Part model, mm, in its own coordinate system. Face numbers are marked on the shaded views. A direction names the side the tool comes from. Round coordinates to 2 decimals unless told otherwise and drop trailing zeros. Loops run counter-clockwise (first coordinate to the right, second up) from the corner with the lowest first, then second, coordinate; pieces in that order, holes last. Notation, with made-up numbers: M -12,-34 L 37,-34 A21 cw 37,-18 Z; hole C 84,4 d3. An arc over 180 degrees is marked long. Answer as CSV lines item,"result". Start each with the question number.
Item 1: Band-saw the part on A-A (y = 47). Give the cut face in (x, z).
Item 2: Which spindle directions (+Z, -Z, +X, -X, +Y, -Y) get a long thin tool onto all of the face, cutting with end or side? Do the marked faces 1, 2 and 3. Say none if no direction does.
Item 3: Band-saw the part on C-C (z = 4.25). Count the separate pieces of the cut face and the enclosed holes in it, and give its area (3 significant figures).
Item 4: Drop flat-ended pins along their axis: pin 1 Ø1.5 at (y, z) = (46.5, 3.5) entering from -X; pin 2 Ø0.8 at (x, y) = (-45, -0.5) entering from +Z; pin 3 Ø0.5 at (y, z) = (48.5, 4) entering from -X; pin 4 Ø1.8 at (x, y) = (-58.66, 30) entering from +Z. Give the stop position or say it passes through.
Item 5: Mould opens along X. For the marked faces 4, 5 and 6 say: pulls with the +X half, pulls with the -X half, needs draft (parallel to the pull), parting line crosses it, or undercut.
Item 6: Wall check: line 1 (Y direction, x = -50, z = 1.25); line 2 (X direction, y = 20, z = 2.7); line 3 (X direction, y = 11.5, z = 2.05). Give the ranges that are in metal, low to high.
Item 7: Band-saw the part on B-B (y = 20). Give the cut face in (x, z).
Autodesk Fusion 360 part; units mm, degrees
sketch "Sketch3" plane through (0, 0, 0) normal (0, 0, 1) x (1, 0, 0)
  circle A0 centre (-50, 25) radius 27.5
  line L0 (-40.5, 45) -> (-40.5, 60)
  line L1 (-59.5, 60) -> (-59.5, 45)
  line L2 (-50, 25) -> (-50, 55)
  circle A1 centre (-50, 25) radius 16.25
  spline S0 degree 2 poles (-59.5, 45) (-50.3564, 40) (-40.5, 45) knots 0 0 0 2.042764 2.042764 2.042764 weights 1 3 1
  dimension "d9" = 55
  dimension "d10" = 32.5
extrude "Extrude3" add sketch "Sketch3" along normal blind 5 contours A0 L0 L1 L2 A1 S0 | A0 L0 L2 S0 | A0 L1 L2 S0 | A1
sketch "Sketch4" plane through (0, 0, 5) normal (0, 0, 1) x (-1, 0, 0)
  circle A0 centre (50, -25) radius 27.5
  line L0 (50, -25) -> (50, -61)
  line L1 (59.5, -45) -> (59.5, -62)
  line L2 (40.5, -62) -> (40.5, -45)
  circle A1 centre (50, -25) radius 16.25
  spline S0 degree 2 poles (59.5, -45) (50, -40) (40.5, -45) knots 0 0 0 2.04267 2.04267 2.04267 weights 1 3 1
  line L3 (82.2534, -45.4687) -> (66.0855, -40.2154)
  spline S1 degree 2 poles (71.9568, -22.1453) (64.2658, -29.6353) (66.0855, -40.2154) knots 0 0 0 2.04267 2.04267 2.04267 weights 1 3 1
  line L4 (71.9568, -22.1453) -> (88.1248, -27.3986)
  line L5 (50, -25) -> (84.238, -36.1246)
  line L6 (79.4337, -0.6503) -> (69.4414, -14.4036)
  spline S2 degree 2 poles (54.07, -3.2357) (58.8168, -12.8647) (69.4414, -14.4036) knots 0 0 0 2.04267 2.04267 2.04267 weights 1 3 1
  line L7 (54.07, -3.2357) -> (64.0624, 10.5176)
  line L8 (50, -25) -> (71.1603, 4.1246)
  line L9 (35.9376, 10.5176) -> (45.93, -3.2357)
  spline S3 degree 2 poles (30.5586, -14.4036) (41.1832, -12.8647) (45.93, -3.2357) knots 0 0 0 2.04267 2.04267 2.04267 weights 1 3 1
  line L10 (30.5586, -14.4036) -> (20.5663, -0.6503)
  line L11 (50, -25) -> (28.8397, 4.1246)
  line L12 (11.8752, -27.3986) -> (28.0432, -22.1453)
  spline S4 degree 2 poles (33.9145, -40.2154) (35.7342, -29.6353) (28.0432, -22.1453) knots 0 0 0 2.04267 2.04267 2.04267 weights 1 3 1
  line L13 (33.9145, -40.2154) -> (17.7466, -45.4687)
  line L14 (50, -25) -> (15.762, -36.1246)
  dimension "d14" = 32.5
  dimension "d21" = 360
extrude "Extrude4" cut sketch "Sketch4" against normal blind 30 contours A0 S1 L4 L5 | A0 L3 S1 L5 | A0 L6 S2 L8 | A0 S2 L7 L8 | A0 L0 L1 S0 | A0 L0 L2 S0 | A0 L12 S4 L14 | A0 S4 L13 L14 | A0 L9 S3 L11 | A0 S3 L10 L11
sketch "Sketch5" plane through (0, 0, 5) normal (0, 0, 1) x (-1, 0, 0)
  line L0 (71.9568, -22.1453) -> (77.4796, -23.9398)
  arc A0 (77.4796, -23.9398) -> (72.8546, -9.7057) centre (50, -25) ccw
  line L1 (72.8546, -9.7057) -> (69.4414, -14.4036)
  spline S0 degree 2 poles (69.4414, -14.4036) (58.8168, -12.8647) (54.07, -3.2357) knots -2.04267 -2.04267 -2.04267 0 0 0 weights 1 3 1
  line L2 (54.07, -3.2357) -> (57.4833, 1.4622)
  arc A1 (57.4833, 1.4622) -> (42.5167, 1.4622) centre (50, -25) ccw
  line L3 (42.5167, 1.4622) -> (45.93, -3.2357)
  spline S1 degree 2 poles (45.93, -3.2357) (41.1832, -12.8647) (30.5586, -14.4036) knots -2.04267 -2.04267 -2.04267 0 0 0 weights 1 3 1
  line L4 (30.5586, -14.4036) -> (27.1454, -9.7057)
  arc A2 (27.1454, -9.7057) -> (22.5204, -23.9398) centre (50, -25) ccw
  line L5 (22.5204, -23.9398) -> (28.0432, -22.1453)
  spline S2 degree 2 poles (28.0432, -22.1453) (35.7342, -29.6353) (33.9145, -40.2154) knots -2.04267 -2.04267 -2.04267 0 0 0 weights 1 3 1
  line L6 (33.9145, -40.2154) -> (28.3918, -42.0098)
  arc A3 (28.3918, -42.0098) -> (40.5, -50.807) centre (50, -25) ccw
  line L7 (40.5, -50.807) -> (40.5, -45)
  spline S3 degree 2 poles (40.5, -45) (50, -40) (59.5, -45) knots -2.04267 -2.04267 -2.04267 0 0 0 weights 1 3 1
  line L8 (59.5, -45) -> (59.5, -50.807)
  arc A4 (59.5, -50.807) -> (71.6082, -42.0098) centre (50, -25) ccw
  line L9 (71.6082, -42.0098) -> (66.0855, -40.2154)
  spline S4 degree 2 poles (66.0855, -40.2154) (64.2658, -29.6353) (71.9568, -22.1453) knots -2.04267 -2.04267 -2.04267 0 0 0 weights 1 3 1
  circle A5 centre (50, -25) radius 10
  circle A6 centre (50, -35) radius 1.5
  circle A7 centre (58.6603, -30) radius 1.5
  circle A8 centre (58.6603, -20) radius 1.5
  circle A9 centre (50, -15) radius 1.5
  circle A10 centre (41.3397, -20) radius 1.5
  circle A11 centre (41.3397, -30) radius 1.5
  circle A12 centre (50, -25) radius 6
  line L10 (50, -25) -> (33.8359, -47.248)
  circle A13 centre (35.5881, -44.8363) radius 1.5
  circle A14 centre (64.4119, -44.8363) radius 1.5
  circle A15 centre (73.319, -17.4232) radius 1.5
  circle A16 centre (50, -0.481) radius 1.5
  circle A17 centre (26.681, -17.4232) radius 1.5
  dimension "d24" = 20
  dimension "d25" = 3
  dimension "d27" = 360
  dimension "d28" = 3
  dimension "d30" = 360
extrude "Extrude5" cut sketch "Sketch5" against normal blind 5 contours A12 | L10 A13 | L10 A13 | A5 A11 | A5 A11 | A5 A6 | A5 A6 | A5 A10 | A5 A10 | A5 A7 | A5 A7 | A5 A9 | A5 A9 | A5 A8 | A5 A8 | A14 | A15 | A16 | A17
sketch "Sketch6" plane through (0, 0, 5) normal (0, 0, 1) x (-1, 0, 0)
  line L0 (71.9568, -22.1453) -> (77.4796, -23.9398)
  arc A0 (77.4796, -23.9398) -> (72.8546, -9.7057) centre (50, -25) ccw
  line L1 (72.8546, -9.7057) -> (69.4414, -14.4036)
  spline S0 degree 2 poles (69.4414, -14.4036) (58.8168, -12.8647) (54.07, -3.2357) knots -2.04267 -2.04267 -2.04267 0 0 0 weights 1 3 1
  line L2 (54.07, -3.2357) -> (57.4833, 1.4622)
  arc A1 (57.4833, 1.4622) -> (42.5167, 1.4622) centre (50, -25) ccw
  line L3 (42.5167, 1.4622) -> (45.93, -3.2357)
  spline S1 degree 2 poles (45.93, -3.2357) (41.1832, -12.8647) (30.5586, -14.4036) knots -2.04267 -2.04267 -2.04267 0 0 0 weights 1 3 1
  line L4 (30.5586, -14.4036) -> (27.1454, -9.7057)
  arc A2 (27.1454, -9.7057) -> (22.5204, -23.9398) centre (50, -25) ccw
  line L5 (22.5204, -23.9398) -> (28.0432, -22.1453)
  spline S2 degree 2 poles (28.0432, -22.1453) (35.7342, -29.6353) (33.9145, -40.2154) knots -2.04267 -2.04267 -2.04267 0 0 0 weights 1 3 1
  line L6 (33.9145, -40.2154) -> (28.3918, -42.0098)
  arc A3 (28.3918, -42.0098) -> (40.5, -50.807) centre (50, -25) ccw
  line L7 (40.5, -50.807) -> (40.5, -45)
  spline S3 degree 2 poles (40.5, -45) (50, -40) (59.5, -45) knots -2.04267 -2.04267 -2.04267 0 0 0 weights 1 3 1
  line L8 (59.5, -45) -> (59.5, -50.807)
  arc A4 (59.5, -50.807) -> (71.6082, -42.0098) centre (50, -25) ccw
  line L9 (71.6082, -42.0098) -> (66.0855, -40.2154)
  spline S4 degree 2 poles (66.0855, -40.2154) (64.2658, -29.6353) (71.9568, -22.1453) knots -2.04267 -2.04267 -2.04267 0 0 0 weights 1 3 1
  circle A5 centre (50, -0.481) radius 1.5
  circle A6 centre (35.5881, -44.8363) radius 1.5
  circle A7 centre (58.6603, -30) radius 1.5
  circle A8 centre (50, -25) radius 6
  circle A9 centre (58.6603, -20) radius 1.5
  circle A10 centre (64.4119, -44.8363) radius 1.5
  circle A11 centre (26.681, -17.4232) radius 1.5
  circle A12 centre (41.3397, -20) radius 1.5
  circle A13 centre (50, -35) radius 1.5
  circle A14 centre (41.3397, -30) radius 1.5
  circle A15 centre (50, -15) radius 1.5
  circle A16 centre (73.319, -17.4232) radius 1.5
  circle A17 centre (50, -25) radius 14
  dimension "d33" = 28
extrude "Extrude6" cut sketch "Sketch6" against normal blind 1.5 contours A17
sketch "Sketch7" plane through (0, 0, 5) normal (0, 0, 1) x (-1, 0, 0)
  circle A0 centre (73.319, -17.4232) radius 1.5
  circle A1 centre (26.681, -17.4232) radius 1.5
  circle A2 centre (64.4119, -44.8363) radius 1.5
  circle A3 centre (35.5881, -44.8363) radius 1.5
  circle A4 centre (50, -0.481) radius 1.5
  line L0 (71.9568, -22.1453) -> (77.4796, -23.9398)
  arc A5 (77.4796, -23.9398) -> (72.8546, -9.7057) centre (50, -25) ccw
  line L1 (72.8546, -9.7057) -> (69.4414, -14.4036)
  spline S0 degree 2 poles (69.4414, -14.4036) (58.8168, -12.8647) (54.07, -3.2357) knots -2.04267 -2.04267 -2.04267 0 0 0 weights 1 3 1
  line L2 (54.07, -3.2357) -> (57.4833, 1.4622)
  arc A6 (57.4833, 1.4622) -> (42.5167, 1.4622) centre (50, -25) ccw
  line L3 (42.5167, 1.4622) -> (45.93, -3.2357)
  spline S1 degree 2 poles (45.93, -3.2357) (41.1832, -12.8647) (30.5586, -14.4036) knots -2.04267 -2.04267 -2.04267 0 0 0 weights 1 3 1
  line L4 (30.5586, -14.4036) -> (27.1454, -9.7057)
  arc A7 (27.1454, -9.7057) -> (22.5204, -23.9398) centre (50, -25) ccw
  line L5 (22.5204, -23.9398) -> (28.0432, -22.1453)
  spline S2 degree 2 poles (28.0432, -22.1453) (35.7342, -29.6353) (33.9145, -40.2154) knots -2.04267 -2.04267 -2.04267 0 0 0 weights 1 3 1
  line L6 (33.9145, -40.2154) -> (28.3918, -42.0098)
  arc A8 (28.3918, -42.0098) -> (40.5, -50.807) centre (50, -25) ccw
  line L7 (40.5, -50.807) -> (40.5, -45)
  spline S3 degree 2 poles (40.5, -45) (50, -40) (59.5, -45) knots -2.04267 -2.04267 -2.04267 0 0 0 weights 1 3 1
  line L8 (59.5, -45) -> (59.5, -50.807)
  arc A9 (59.5, -50.807) -> (71.6082, -42.0098) centre (50, -25) ccw
  line L9 (71.6082, -42.0098) -> (66.0855, -40.2154)
  spline S4 degree 2 poles (66.0855, -40.2154) (64.2658, -29.6353) (71.9568, -22.1453) knots -2.04267 -2.04267 -2.04267 0 0 0 weights 1 3 1
  circle A10 centre (50, -25) radius 14
  line L10 (61, -48) -> (39, -48)
  line L11 (50, -25) -> (50, -48)
  line L12 (61, -49) -> (39, -49)
  line L13 (39, -49) -> (39, -48)
  line L14 (61, -49) -> (61, -48)
  line L15 (75.2735, -21.6458) -> (68.4751, -42.569)
  line L16 (76.2245, -21.9548) -> (75.2735, -21.6458)
  line L17 (76.2245, -21.9548) -> (69.4262, -42.878)
  line L18 (69.4262, -42.878) -> (68.4751, -42.569)
  line L19 (54.6199, 0.073) -> (72.4182, -12.8582)
  line L20 (55.2077, 0.882) -> (54.6199, 0.073)
  line L21 (55.2077, 0.882) -> (73.006, -12.0492)
  line L22 (73.006, -12.0492) -> (72.4182, -12.8582)
  line L23 (27.5818, -12.8582) -> (45.3801, 0.073)
  line L24 (26.994, -12.0492) -> (27.5818, -12.8582)
  line L25 (26.994, -12.0492) -> (44.7923, 0.882)
  line L26 (44.7923, 0.882) -> (45.3801, 0.073)
  line L27 (31.5249, -42.569) -> (24.7265, -21.6458)
  line L28 (30.5738, -42.878) -> (31.5249, -42.569)
  line L29 (30.5738, -42.878) -> (23.7755, -21.9548)
  line L30 (23.7755, -21.9548) -> (24.7265, -21.6458)
  dimension "d37" = 360
extrude "Extrude7" cut sketch "Sketch7" against normal blind 1.5 contours L0 L15 L16 L17 | L9 L15 L17 L18 | L1 L19 L21 L22 | L2 L19 L20 L21 | L8 L10 L12 L14 | L7 L10 L12 L13 | L3 L23 L25 L26 | L4 L23 L24 L25 | L6 L27 L28 L29 | L5 L27 L29 L30
sketch "Sketch1" plane through (0, 0, 0) normal (0, 0, 1) x (1, 0, 0)
  circle A0 centre (-75, 50) radius 40
extrude "Extrude1" [suppressed]
sketch "Sketch2" plane through (0, 0, 40) normal (0, 0, 1) x (-1, 0, 0)
  circle A0 centre (75, -50) radius 40
  circle A1 centre (75, -50) radius 30
  line L0 (75, -50) -> (56.4216, -73.5551)
  line L1 (75, -50) -> (93.5784, -73.5551)
  line L2 (75, -50) -> (93.5784, -26.4449)
  line L3 (56.4216, -26.0914) -> (75, -50)
extrude "Extrude2" [suppressed]
fillet "Fillet1" [suppressed]
fillet "Fillet2" [suppressed]
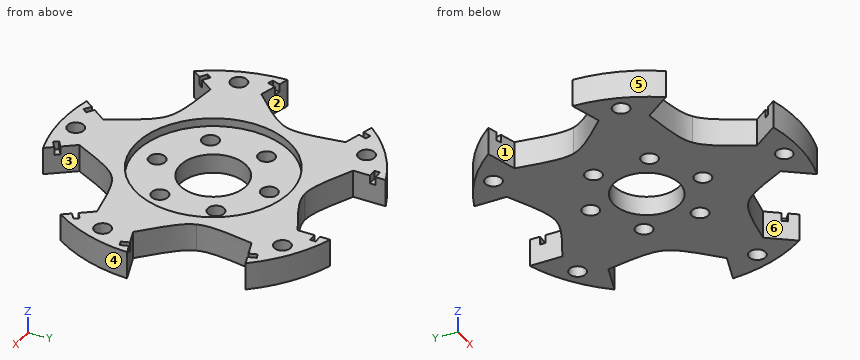
Answer block:
1,outline,"M -66.5,0 L -59.5,0 L -59.5,5 L -66.5,5 Z; M -40.5,0 L -33.5,0 L -33.5,5 L -40.5,5 Z"
2,face 1,"+Z, -Z, -X"
2,face 2,"+Z, -Z, +Y"
2,face 3,"+Z, -Z, +X"
3,separate pieces,"1"
3,enclosed holes,"6"
3,area,"838 mm^2"
4,pin 1,"stops at x = -68.05"
4,pin 2,"stops at z = 5"
4,pin 3,"stops at x = -64.69"
4,pin 4,"passes through"
5,face 4,"pulls with the +X half"
5,face 5,"pulls with the -X half"
5,face 6,"undercut"
6,line 1,"y = -2.5 to -1.02, 1.98 to 13.5, 16.5 to 19, 31 to 33.5, 36.5 to 41.25"
6,line 2,"x = -77.04 to -60.16, -57.16 to -53.32, -46.68 to -42.84, -39.84 to -22.96"
6,line 3,"x = -73.96 to -71.55, -59.11 to -40.89, -28.45 to -26.04"
7,outline,"M -77.04,0 L -60.16,0 L -60.16,3.5 L -63.08,3.5 L -63.08,5 L -77.04,5 Z; M -57.16,0 L -53.32,0 L -53.32,3.5 L -57.16,3.5 Z; M -46.68,0 L -42.84,0 L -42.84,3.5 L -46.68,3.5 Z; M -39.84,0 L -22.96,0 L -22.96,5 L -36.92,5 L -36.92,3.5 L -39.84,3.5 Z"
